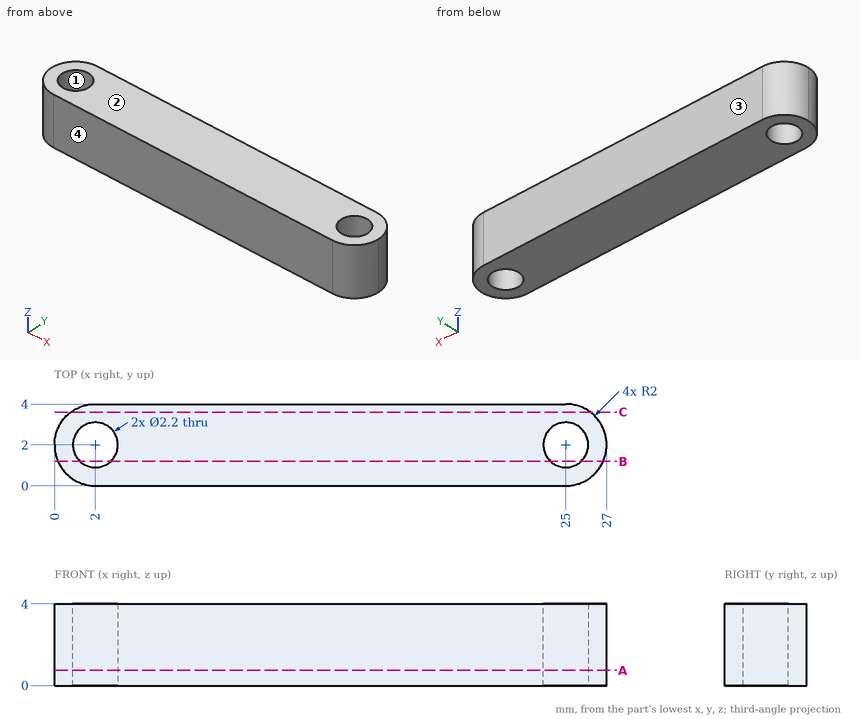
Here's the drawing with two shaded views (mm, measured from the low corner). I have some questions. Coordinates: 2 decimals unless noted, no trailing zeros. Write each loop counter-clockwise with the first axis right and the second up, starting at its lowest first coordinate (ties: lowest second). Pieces come first, ordered by that corner, then holes. Notation, with made-up numbers: (-11, -11.5) -> (37, -11.5) arc R20 ccw to (37, 25.5) -> close; hole circle Ø9 at (27.5, -10.5). An arc over 180 degrees is marked (long way). Answer as CSV lines item,"result".
1) Will this pin go through, and if not, where does the flat tip stop? P1, Ø1.5, axis at x = 8.5, z = 2.5, coming from the -Y side.
Check result:
P1,"y = 0"
2) If we section it at A-A on z = 0.75: Count the separate pieces of the cut face and the enclosed holes in it.
Check result:
separate pieces,"1"
enclosed holes,"2"
3) If we mould it in two halves opening along Y, with no side actions, what happens to the marked faces 1, 2, 3 and 4? For each: +Y half, -Y half, draft (parallel to the pull), parting line (faces both ways), or undercut.
Check result:
face 1,"undercut"
face 2,"draft"
face 3,"+Y half"
face 4,"-Y half"
4) If I drill on line 1 (Y direction, x = 2, z = 1.2); line 2 (X direction, y = 2.5, z = 3.2); line 3 (X direction, y = 1.8, z = 1.1), over which ranges is the centre line in solid material (lowest first)? Write a range as from..to.
Check result:
line 1,"0..0.9, 3.1..4"
line 2,"0.06..1.02, 2.98..24.02, 25.98..26.94"
line 3,"0.01..0.92, 3.08..23.92, 26.08..26.99"
5) If we section it at C-C on y = 3.6: Please give me the cut outline in (x, z).
Check result:
outline,"(0.8, 0) -> (26.2, 0) -> (26.2, 4) -> (0.8, 4) -> close"
6) If we section it at B-B on y = 1.2: Please give me the cut outline in (x, z) (3 decimals), then the cut area to 3 significant figures.
Check result:
outline,"(0.167, 0) -> (1.245, 0) -> (1.245, 4) -> (0.167, 4) -> close; (2.755, 0) -> (24.245, 0) -> (24.245, 4) -> (2.755, 4) -> close; (25.755, 0) -> (26.833, 0) -> (26.833, 4) -> (25.755, 4) -> close"
area,"94.6 mm²"
